```python
from build123d import *

# Parameters (mm, degrees)
BOSS_EXTRUDE1_DEPTH = 20
SKETCH2_R           = 7.5
BOSS_EXTRUDE2_DEPTH = 30


with BuildPart() as part:
    # Sketch1 → Boss-Extrude1 (new body)
    with BuildSketch(Plane(origin=(0, 0, 0), x_dir=(1, 0, 0), z_dir=(0, 1, 0))):
        with BuildLine():
            Line((0, -25), (30, -25))
            Line((30, -25), (30, 25))
            Line((30, 25), (0, 25))
            ThreePointArc((0, 25), (-25, 0), (0, -25))
        make_face()
        with BuildLine():
            Line((3.75, 6.5), (2.47446787, 15.356382884))
            ThreePointArc((2.47446787, 15.356382884), (0, 17.5), (-2.47446787, 15.356382884))
            Line((-2.47446787, 15.356382884), (-3.75, 6.5))
            Line((-3.75, 6.5), (-3.754165125, 6.497595264))
            Line((-3.754165125, 6.497595264), (-12.061783753, 9.821143478))
            ThreePointArc((-12.061783753, 9.821143478), (-15.155444566, 8.75), (-14.536251623, 5.535239406))
            Line((-14.536251623, 5.535239406), (-7.504165125, 0.002404736))
            Line((-7.504165125, 0.002404736), (-7.504165125, -0.002404736))
            Line((-7.504165125, -0.002404736), (-14.536251623, -5.535239406))
            ThreePointArc((-14.536251623, -5.535239406), (-15.155444566, -8.75), (-12.061783753, -9.821143478))
            Line((-12.061783753, -9.821143478), (-3.754165125, -6.497595264))
            Line((-3.754165125, -6.497595264), (-3.75, -6.5))
            Line((-3.75, -6.5), (-2.47446787, -15.356382884))
            ThreePointArc((-2.47446787, -15.356382884), (0, -17.5), (2.47446787, -15.356382884))
            Line((2.47446787, -15.356382884), (3.75, -6.5))
            Line((3.75, -6.5), (3.754165125, -6.497595264))
            Line((3.754165125, -6.497595264), (12.061783753, -9.821143478))
            ThreePointArc((12.061783753, -9.821143478), (15.155444566, -8.75), (14.536251623, -5.535239406))
            Line((14.536251623, -5.535239406), (7.504165125, -0.002404736))
            Line((7.504165125, -0.002404736), (7.504165125, 0.002404736))
            Line((7.504165125, 0.002404736), (14.536251623, 5.535239406))
            ThreePointArc((14.536251623, 5.535239406), (15.155444566, 8.75), (12.061783753, 9.821143478))
            Line((12.061783753, 9.821143478), (3.754165125, 6.497595264))
            Line((3.754165125, 6.497595264), (3.75, 6.5))
        make_face(mode=Mode.SUBTRACT)
    extrude(amount=BOSS_EXTRUDE1_DEPTH)

    # Sketch2 → Boss-Extrude2 (add)
    with BuildSketch(Plane(origin=(0, 20, 0), x_dir=(1, 0, 0), z_dir=(0, 1, 0))):
        with BuildLine():
            Line((0, 25), (30, 25))
            Line((30, 25), (30, -25))
            Line((30, -25), (0, -25))
            ThreePointArc((0, -25), (-25, 0), (0, 25))
        make_face()
        with Locations(Location((0, 0, 0), (0, 0, 270))):
            Circle(SKETCH2_R, mode=Mode.SUBTRACT)
    extrude(amount=BOSS_EXTRUDE2_DEPTH)


solid = part.part
```
CAD build for the part. Positions are in the model's coordinates, mm. A direction names the side the tool comes from. Round coordinates to 2 decimals unless told otherwise and drop trailing zeros. Loops run counter-clockwise (first coordinate to the right, second up) from the corner with the lowest first, then second, coordinate; pieces in that order, holes last. Notation, with made-up numbers: M 82,81.25 L 93,81.25 A27 ccw 93,107.25 Z; hole C -3,-31.75 d4. An arc over 180 degrees is marked long. Return JSON: item names as keys, results as strings. Group by question number.
(1) Saw through at D-D, the plane x = 10. List the corners of the cut face in (y, z).
(2) Drop flat-ended pins along their axis: P1, Ø10, axis at x = 10, z = 2.5, coming from the -Y side; P2, Ø5, axis at y = 5, z = -3.5, coming from the -X side. Give the stop position or say it passes through.
(3) Tool access for faces 5 (the flat face through (30, 25, 0)), 6 (the flat face through (-3.1, 9.9, -11)): list every direction of +Z, -Z, +X, -X, +Y, -Y with a clear straight run to the whole face (end or side of a thin tool).
(4) Wall check: probe 1 along X at (y, z) = (40, 0); probe 2 along Y at (x, z) = (-7.5, 2.5); probe 3 along Z at (x, y) = (-1, 18). Give the ranges that are in metal, low to high. Write a range as [from, to].
(5) Saw through at B-B, the plane x = -5. List the corners of the cut face in (y, z), and give its area (3 significant figures).
(6) Saw through at C-C, the plane z = -13. List the corners of the cut face in (x, y).
(7) Mould opens along Z. For faces 1 (the cylindrical face through (-24.994, 24.65, 0.55)), 2 (the cylindrical face through (0, 9.9, 17.5)), 3 (the cylindrical face through (15.13, 9.86, 8.79)), 4 (the flat face through (15, 25, -25)) say: +Z half, -Z half, draft (parallel to the pull), parting line (faces both ways), or undercut.
Answer list:
{
 "1": {"outline": "M 0,-25 L 50,-25 L 50,25 L 0,25 L 0,9 L 20,9 L 20,1.97 L 0,1.97 L 0,-1.97 L 20,-1.97 L 20,-9 L 0,-9 Z"},
 "2": {"P1": "y = 0", "P2": "x = -24.98"},
 "3": {"face 5": "+Z, -Z, +X, +Y, -Y", "face 6": "-Y"},
 "4": {"probe 1": "[-25, -7.5], [7.5, 30]", "probe 2": "[20, 50]", "probe 3": "[-24.98, -17.29], [17.29, 24.98]"},
 "5": {"outline": "M 0,-24.49 L 50,-24.49 L 50,-5.59 L 20,-5.59 L 20,-7 L 0,-7 Z; M 0,7 L 20,7 L 20,5.59 L 50,5.59 L 50,24.49 L 0,24.49 Z", "area": "1,830 mm2"},
 "6": {"outline": "M -21.35,0 L -2.81,0 L -2.81,20 L 2.81,20 L 2.81,0 L 30,0 L 30,50 L -21.35,50 Z"},
 "7": {"face 1": "parting line", "face 2": "undercut", "face 3": "undercut", "face 4": "-Z half"}
}
